Here's how the part is built. I have some questions about the finished solid (model axes, mm). A direction names the side the tool comes from. Give positions to 0.01 mm unless a question says otherwise; leave off trailing zeros. Order: outer loops, then holes, each group sorted by start corner. A loop starts at its lowest first (then second) coordinate and runs counter-clockwise, first axis right, second up.
from build123d import *

# Parameters (mm, degrees)
SKETCH2_W      = 31.1404
SKETCH2_H      = 76.2
EXTRUDE1_DEPTH = 2.0066
SKETCH3_W      = 22.0472
SKETCH3_H      = 67.1068
EXTRUDE2_DEPTH = 2.0066
SKETCH4_W      = 26.0604
SKETCH4_H      = 71.12
EXTRUDE3_DEPTH = 2.0066
SKETCH5_W      = 31.1404
SKETCH5_H      = 7
EXTRUDE4_DEPTH = 2.25


with BuildPart() as part:
    # Sketch2 → Extrude1 (new body)
    with BuildSketch(Plane.XY):
        Rectangle(SKETCH2_W, SKETCH2_H)
    extrude(amount=EXTRUDE1_DEPTH)

    # Sketch3 → Extrude2 (add)
    with BuildSketch(Plane.XY.offset(2.0066)):
        Rectangle(SKETCH3_W, SKETCH3_H)
    extrude(amount=EXTRUDE2_DEPTH)

    # Sketch4 → Extrude3 (add)
    with BuildSketch(Plane.XY.offset(4.0132)):
        Rectangle(SKETCH4_W, SKETCH4_H)
    extrude(amount=EXTRUDE3_DEPTH)

    # Sketch5 → Extrude4 (add)
    with BuildSketch(Plane(origin=(0, 0, 0), x_dir=(-1, 0, 0), z_dir=(0, 0, -1))):
        with Locations((0, -36.6)):
            Rectangle(SKETCH5_W, SKETCH5_H)
    extrude(amount=EXTRUDE4_DEPTH)


solid = part.part
Q1. Thinking about a two-plate mould opening in Z: for faces 5 (the face through (11.024, 0, 3)), 6 (the face through (0, -37, -2.25)), 7 (the face through (-15.57, -2, 1)), which applies, released by +Z, released by -Z, zero draft, split by the parting line, or undercut?
Filled sheet:
face 5: undercut
face 6: released by -Z
face 7: zero draft
Q2. If we section it at C-C on z = 4.75: List the corners of the cut face in (x, y) for me.
Filled sheet:
outline: (-13.03, -35.56) - (13.03, -35.56) - (13.03, 35.56) - (-13.03, 35.56) - close
Q3. If we section it at B-B on x = -3: List the corners of the cut face in (y, z) for me.
Filled sheet:
outline: (-40.1, -2.25) - (-33.1, -2.25) - (-33.1, 0) - (38.1, 0) - (38.1, 2.01) - (33.55, 2.01) - (33.55, 4.01) - (35.56, 4.01) - (35.56, 6.02) - (-35.56, 6.02) - (-35.56, 4.01) - (-33.55, 4.01) - (-33.55, 2.01) - (-38.1, 2.01) - (-38.1, 0) - (-40.1, 0) - close
Q4. I need wall thicknesses on L1, parallel to Z at x = 14, y = -22; L2, parallel to Z at x = 3.5, y = -25.5; L3, parallel to X at y = -11.5, z = 5.75. Which ranges of each line are inside material? Lowest first, please.
Filled sheet:
L1: z = 0 to 2.01
L2: z = 0 to 6.02
L3: x = -13.03 to 13.03
Q5. For faces 1 (the face through (-12, 3, 4.013)), 2 (the face through (0, -38.1, 1)), 3 (the face through (0, 33.553, 3)), 4 (the face through (-11.024, 0, 3)), which set-ups out of +Z, -Z, +X, -X, +Y, -Y let a thin tool reach every point of the face, with its end or its side?
Filled sheet:
face 1: none
face 2: +Z, +X, -X, -Y
face 3: +X, -X, +Y
face 4: -X, +Y, -Y
Q6. If we section it at D-D on z = -0.75: List the corners of the cut face in (x, y) for me.
Filled sheet:
outline: (-15.57, -40.1) - (15.57, -40.1) - (15.57, -33.1) - (-15.57, -33.1) - close
Q7. If we section it at A-A on y = -20: List the corners of the cut face in (x, z) for me, plus the area to 3 significant figures.
Filled sheet:
outline: (-15.57, 0) - (15.57, 0) - (15.57, 2.01) - (11.02, 2.01) - (11.02, 4.01) - (13.03, 4.01) - (13.03, 6.02) - (-13.03, 6.02) - (-13.03, 4.01) - (-11.02, 4.01) - (-11.02, 2.01) - (-15.57, 2.01) - close
area: 159 mm2
Q8. I'm going to push flat-ended pins straight in: P1, Ø8, axis at x = -8, y = 18, coming from the -Z side; P2, Ø2, axis at x = -0.5, z = 3.5, coming from the +Y side; P3, Ø2, axis at x = -0.5, y = -38.5, coming from the +Z side. Where does each tip first touch, or does it pass through?
Filled sheet:
P1: stops at z = 0
P2: stops at y = 35.56
P3: stops at z = 2.01
